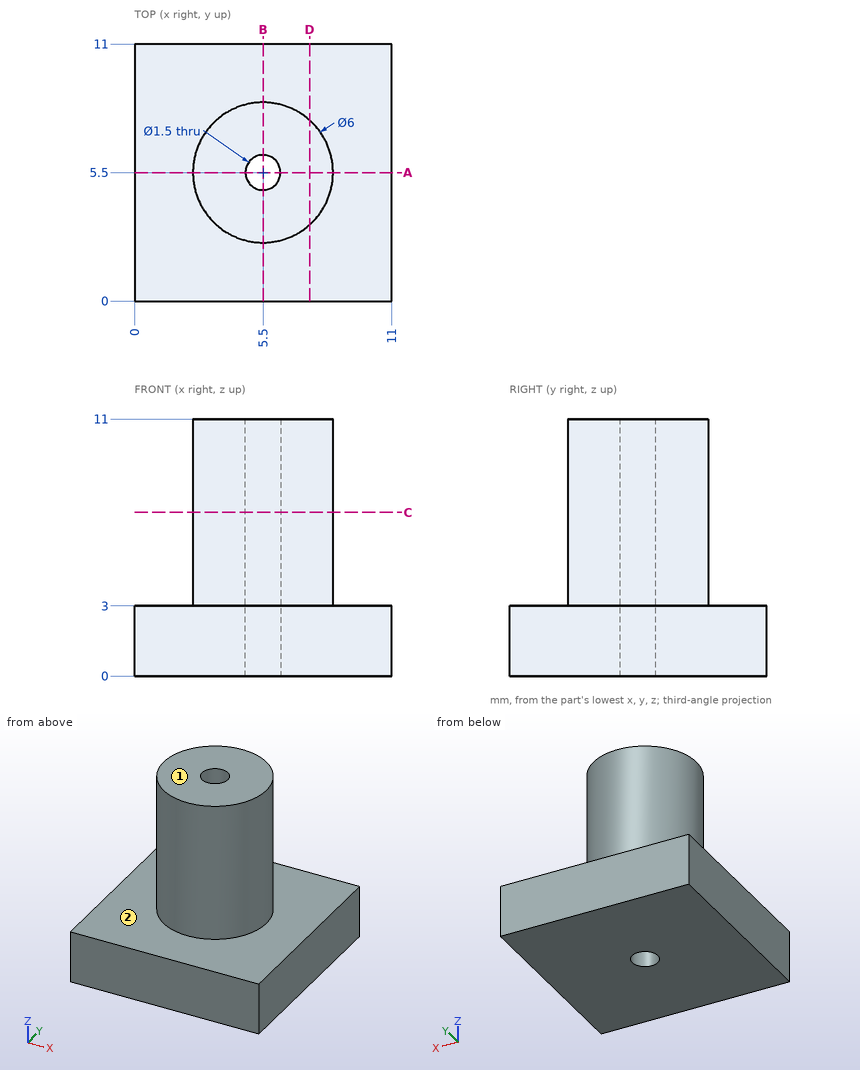
Design review of the part shown in the three views and the two pictorial views. Dimensions are in mm from the part's minimum x, y and z. A direction names the side the tool comes from. Give positions to 0.01 mm unless a question says otherwise; leave off trailing zeros. Loops run counter-clockwise (first coordinate to the right, second up) from the corner with the lowest first, then second, coordinate; pieces in that order, holes last. Notation, with made-up numbers: (48.5, 25.5) -> (59.5, 25.5) arc R31 ccw to (59.5, 64.5) -> close; hole circle Ø4 at (-39, 52). An arc over 180 degrees is marked (long way). One line per question, with ' | ' between items.
1) To check wall thickness, follow probe 1 along Y at (x, z) = (5.5, 4.5); probe 2 along Z at (x, y) = (5.25, 9); probe 3 along Y at (x, z) = (5, 10). State the ranges of each line that lie inside material, in increasing order.
Resolved:
probe 1: y = 2.5 to 4.75, 6.25 to 8.5 | probe 2: z = 0 to 3 | probe 3: y = 2.54 to 4.94, 6.06 to 8.46
2) For the marked faces 1 and 2, list the 3-axis set-ups (+Z, -Z, +X, -X, +Y, -Y) from which the entire face can be reached by the end or side of a thin tool; tool diameter is ignored.
Resolved:
face 1: +Z, +X, -X, +Y, -Y | face 2: +Z
3) We need section D-D (x = 7.5). Write out the cut boundary in (y, z).
Resolved:
outline: (0, 0) -> (11, 0) -> (11, 3) -> (7.74, 3) -> (7.74, 11) -> (3.26, 11) -> (3.26, 3) -> (0, 3) -> close
4) Insertion check: pin 1 Ø4 at (x, z) = (6.5, 8) entering from -Y; pin 2 Ø1 at (x, z) = (1, 5.5) entering from +Y. Each pin has a flat end and moves straight along its axis. Give the tip position at first contact, or say it passes through.
Resolved:
pin 1: stops at y = 2.5 | pin 2: passes through
5) We need section A-A (y = 5.5). Write out the cut boundary in (x, z).
Resolved:
outline: (0, 0) -> (4.75, 0) -> (4.75, 11) -> (2.5, 11) -> (2.5, 3) -> (0, 3) -> close; (6.25, 0) -> (11, 0) -> (11, 3) -> (8.5, 3) -> (8.5, 11) -> (6.25, 11) -> close
6) We need section C-C (z = 7). Write out the cut boundary in (x, y).
Resolved:
outline: circle Ø6 at (5.5, 5.5); hole circle Ø1.5 at (5.5, 5.5)
